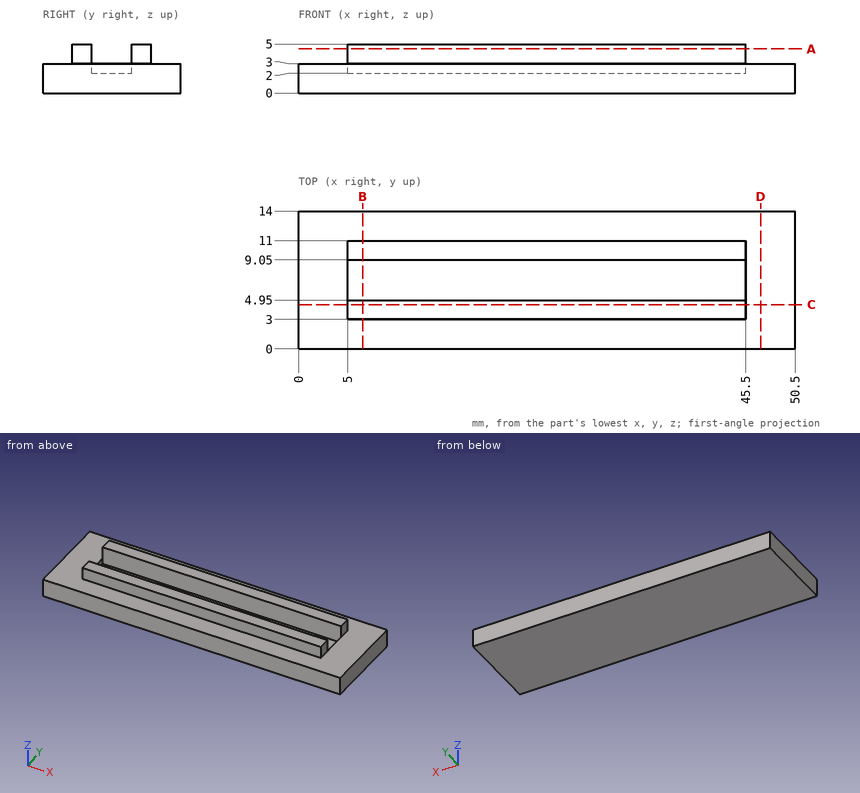
Source: three-view drawing plus pictorial views. Frame: mm from the lowest corner of the part. Round coordinates to 2 decimals unless told otherwise and drop trailing zeros. Order: outer loops, then holes, each group sorted by start corner. A loop starts at its lowest first (then second) coordinate and runs counter-clockwise, first axis right, second up. Notation, with made-up numbers: (21, 32.25) -> (56, 32.25) arc R6 ccw to (56, 39.25) -> close; hole circle Ø10 at (-2.75, 88). An arc over 180 degrees is marked (long way). Use one line per item in the form item = value. Start each with the question number.
1. Pin query (flat end, axial travel): pin 1 Ø1.5 at (x, z) = (28, 3) entering from -Y; pin 2 Ø0.6 at (y, z) = (9.5, 4) entering from +X; pin 3 Ø0.6 at (y, z) = (4, 4) entering from -X; pin 4 Ø1.2 at (x, y) = (16.5, 6.5) entering from +Z. Return the tip coordinate at first contact, or that it passes through.
2. Cut plane A-A (z = 4.5). Return the cut outline in (x, y).
3. Cut plane C-C (y = 4.5). Return the cut outline in (x, z).
4. Line query: probe 1 along Y at (x, z) = (42.5, 4); probe 2 along Y at (x, z) = (9, 2.25); probe 3 along X at (y, z) = (7.5, 2.05). Output: solid intervals per line, ascending.
5. Cut plane D-D (x = 47). Return the cut outline in (y, z).
6. Cut plane B-B (x = 6.5). Return the cut outline in (y, z).
Solution:
q1.pin_1 = 0
q1.pin_2 = 45.5
q1.pin_3 = 5
q1.pin_4 = 2
q2.outline = (5, 3) -> (45.5, 3) -> (45.5, 4.95) -> (5, 4.95) -> close; (5, 9.05) -> (45.5, 9.05) -> (45.5, 11) -> (5, 11) -> close
q3.outline = (0, 0) -> (50.5, 0) -> (50.5, 3) -> (45.5, 3) -> (45.5, 5) -> (5, 5) -> (5, 3) -> (0, 3) -> close
q4.probe_1 = 3 to 4.95, 9.05 to 11
q4.probe_2 = 0 to 4.95, 9.05 to 14
q4.probe_3 = 0 to 5, 45.5 to 50.5
q5.outline = (0, 0) -> (14, 0) -> (14, 3) -> (0, 3) -> close
q6.outline = (0, 0) -> (14, 0) -> (14, 3) -> (11, 3) -> (11, 5) -> (9.05, 5) -> (9.05, 2) -> (4.95, 2) -> (4.95, 5) -> (3, 5) -> (3, 3) -> (0, 3) -> close
